Autodesk Fusion 360 part; units mm, degrees
sketch "Sketch1" plane through (0, 0, 0) normal (0, 0, 1) x (1, 0, 0)
  circle A0 centre (0, 0) radius 67.8
  circle A1 centre (0, 0) radius 50
  line L0 (-150, 40) -> (-126.1943, 40)
  line L1 (-150, -40) -> (-126.1943, -40)
  line L2 (150, 40) -> (126.1943, 40)
  line L3 (150, -40) -> (126.1943, -40)
  arc A2 (-38.6309, -64.2857) -> (38.6309, -64.2857) centre (0, 0) ccw
  arc A3 (38.6309, 64.2857) -> (-38.6309, 64.2857) centre (0, 0) ccw
  line L4 (-172.9129, 10) -> (-188.7298, 10)
  line L5 (-172.9129, -10) -> (-188.7298, -10)
  arc A4 (-172.9129, -10) -> (-172.9129, 10) centre (-150, 0) ccw
  arc A5 (-150, 40) -> (-188.7298, 10) centre (-150, 0) ccw
  arc A6 (-188.7298, -10) -> (-150, -40) centre (-150, 0) ccw
  line L6 (188.7298, 10) -> (172.9129, 10)
  line L7 (188.7298, -10) -> (172.9129, -10)
  arc A7 (172.9129, 10) -> (172.9129, -10) centre (150, 0) ccw
  arc A8 (150, -40) -> (188.7298, -10) centre (150, 0) ccw
  arc A9 (188.7298, 10) -> (150, 40) centre (150, 0) ccw
  arc A10 (-126.1943, 40) -> (-38.6309, 64.2857) centre (-126.1943, 210) ccw
  arc A11 (-38.6309, -64.2857) -> (-126.1943, -40) centre (-126.1943, -210) ccw
  arc A12 (38.6309, 64.2857) -> (126.1943, 40) centre (126.1943, 210) ccw
  arc A13 (126.1943, -40) -> (38.6309, -64.2857) centre (126.1943, -210) ccw
  dimension "d1" = 135.6
  dimension "d2" = 100
  dimension "d3" = 50
  dimension "d4" = 50
  dimension "d5" = 150
  dimension "d6" = 150
  dimension "d7" = 150
  dimension "d8" = 80
  dimension "d9" = 80
  dimension "d16" = 170
  dimension "d17" = 170
  dimension "d18" = 170
extrude "Extrude1" add sketch "Sketch1" along normal blind 20 contours L0 L1 L2 L3 A2 A3 L4 L5 A4 A5 A6 L6 L7 A7 A8 A9 A10 A11 A12 A13
extrude "Extrude2" add sketch "Sketch1" along normal blind 10 contours A0
Here's how the part is built. I have some questions about the finished solid (model axes, mm). A direction names the side the tool comes from. Round coordinates to 2 decimals unless told otherwise and drop trailing zeros. Order: outer loops, then holes, each group sorted by start corner. A loop starts at its lowest first (then second) coordinate and runs counter-clockwise, first axis right, second up. Notation, with made-up numbers: M 13.25,71.25 L 25.25,71.25 A24 cw 25.25,87.25 Z; hole C 84,-10.5 d9. An arc over 180 degrees is marked long. Answer in a Markdown table with one row per item.
Item 1: Imagine slicing it at A-A, the plane y = 0. Write out the boundary of the cut face in (x, z), and give its area (3 significant figures).
A:
| item | result |
|---|---|
| outline | M -125,0 L -50,0 L -50,10 L -67.8,10 L -67.8,20 L -125,20 Z; M 50,0 L 125,0 L 125,20 L 67.8,20 L 67.8,10 L 50,10 Z |
| area | 2,640 mm2 |
Item 2: Imagine slicing it at B-B, the plane x = 0. Write out the boundary of the cut face in (y, z), and give its area (3 significant figures).
A:
| item | result |
|---|---|
| outline | M -75,0 L -50,0 L -50,10 L -67.8,10 L -67.8,20 L -75,20 Z; M 50,0 L 75,0 L 75,20 L 67.8,20 L 67.8,10 L 50,10 Z |
| area | 644 mm2 |
Item 3: Imagine slicing it at D-D, the plane y = 16.5. Write out the boundary of the cut face in (x, z), and give its area (3 significant figures).
A:
| item | result |
|---|---|
| outline | M -186.44,0 L -168.78,0 L -168.78,20 L -186.44,20 Z; M -131.22,0 L -47.2,0 L -47.2,10 L -65.76,10 L -65.76,20 L -131.22,20 Z; M 47.2,0 L 131.22,0 L 131.22,20 L 65.76,20 L 65.76,10 L 47.2,10 Z; M 168.78,0 L 186.44,0 L 186.44,20 L 168.78,20 Z |
| area | 3,700 mm2 |
Item 4: If I drill on L1, parallel to Y at x = -150, z = 15.25; L2, parallel to X at y = 1.5, z = 11; L3, parallel to Y at x = 2, z = 12.5, over which ranges is the centre line in solid material (lowest first)? Write a range as from..to.
A:
| item | result |
|---|---|
| L1 | y = -40..-25, 25..40 |
| L2 | x = -125.05..-67.78, 67.78..125.05 |
| L3 | y = -74.97..-67.77, 67.77..74.97 |
Item 5: For faces 4 (the face through (138, -40, 10)), 5 (the face through (-138, 40, 10)), 6 (the face through (-49.971, -45.822, 14.93)), 7 (the face through (-181, -10, 10)), 8 (the face through (181, 10, 10)), which set-ups out of +Z, -Z, +X, -X, +Y, -Y let a thin tool reach every point of the face, with its end or its side?
A:
| item | result |
|---|---|
| face 4 | +Z, -Z, +X, -Y |
| face 5 | +Z, -Z, -X, +Y |
| face 6 | +Z |
| face 7 | +Z, -Z, -X |
| face 8 | +Z, -Z, +X |
Item 6: I'm going to push flat-ended pins straight in: pin 1 (8 mm diameter, centred on x = 180, z = 12.5, fed in from -Y); pin 2 (3 mm diameter, centred on y = -20, z = 14.5, fed in from -X); pin 3 (6 mm diameter, centred on x = -59.5, z = 14, fed in from -Y); pin 4 (12 mm diameter, centred on x = 56, y = -38, fed in from -Z). Where does each tip first touch, or does it pass through?
A:
| item | result |
|---|---|
| pin 1 | stops at y = -30.4 |
| pin 2 | stops at x = -185.46 |
| pin 3 | stops at y = -54.94 |
| pin 4 | stops at z = 0 |
Item 7: Imagine slicing it at C-C, the plane z = 14.75. Write out the boundary of the cut face in (x, y), and give its area (3 significant figures).
A:
| item | result |
|---|---|
| outline | M -188.73,-10 A40 ccw -150,-40 L -126.19,-40 A170 cw -38.63,-64.29 A75 ccw 38.63,-64.29 A170 cw 126.19,-40 L 150,-40 A40 ccw 188.73,-10 L 172.91,-10 A25 cw long 172.91,10 L 188.73,10 A40 ccw 150,40 L 126.19,40 A170 cw 38.63,64.29 A75 ccw -38.63,64.29 A170 cw -126.19,40 L -150,40 A40 ccw -188.73,10 L -172.91,10 A25 cw long -172.91,-10 Z; hole C 0,0 d135.6 |
| area | 17,700 mm2 |
Item 8: Thinking about a two-plate mould opening in X: for faces 1 (the face through (174, 32, 10)), 2 (the face through (-57, 39, 20)), 3 (the face through (-5, -50, 10)), which applies, +X half, -X half, draft (parallel to the pull), parting line (faces both ways), or undercut?
A:
| item | result |
|---|---|
| face 1 | +X half |
| face 2 | draft |
| face 3 | undercut |
